Job drawing, mm, ordinate dimensions from the low corner. One solid piece. A direction names the side the tool comes from. Give positions to 0.01 mm unless a question says otherwise; leave off trailing zeros. Loops run counter-clockwise (first coordinate to the right, second up) from the corner with the lowest first, then second, coordinate; pieces in that order, holes last. Notation, with made-up numbers: M -8.75,-38.5 L 18.25,-38.5 A18 ccw 18.25,-5.5 Z; hole C 11.5,86.5 d7. An arc over 180 degrees is marked long. Put each result on its own line as item: value.
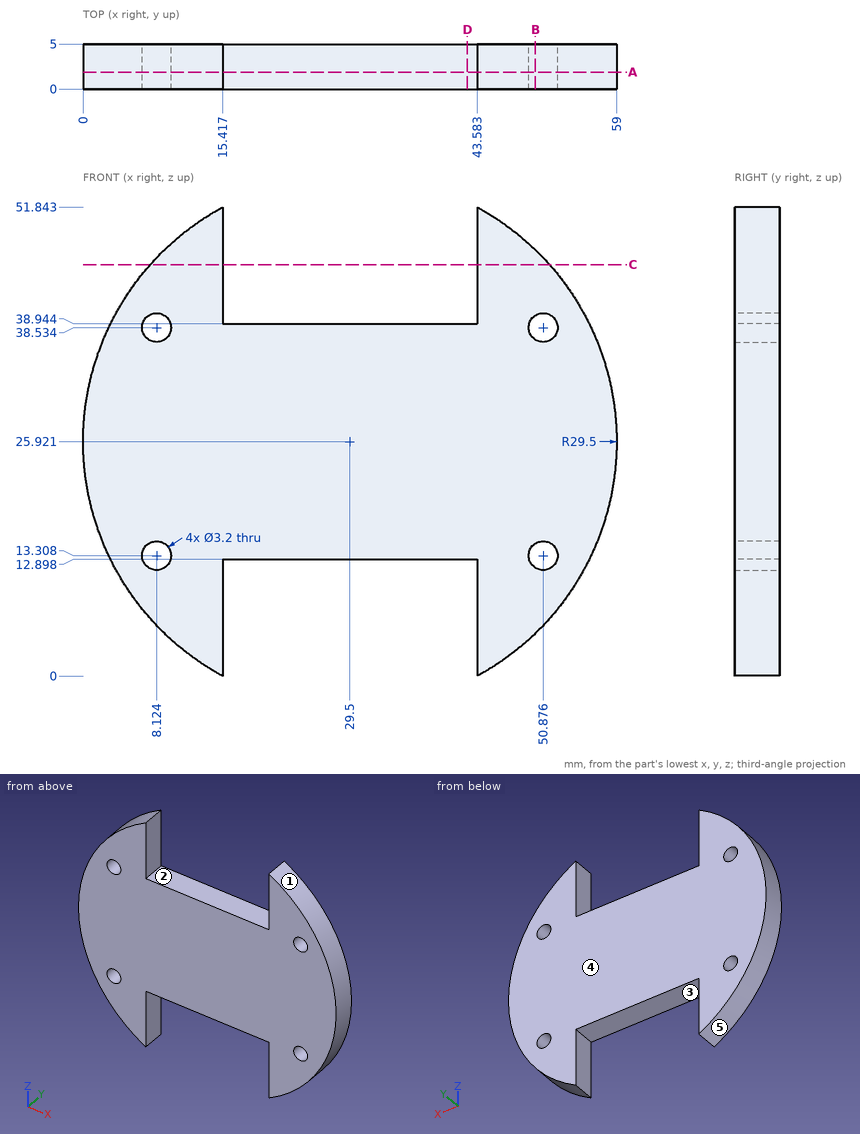
Q1. Probe line 1 (X direction, y = 0.75, z = 13) (1 decimal); line 2 (Z direction, x = 7, y = 2.5) (1 decimal); line 3 (X direction, y = 1.9, z = 12.5) (1 decimal). List the from-to ranges inside material, lowest first. Write a range as from..to.
Here are the results:
line 1: 3..6.6, 9.7..49.3, 52.4..56
line 2: 6.8..12.2, 14.4..37.4, 39.7..45
line 3: 3.2..6.7, 9.5..15.4, 43.6..49.5, 52.3..55.8
Q2. Drop flat-ended pins along their axis: pin 1 Ø2.5 at (y, z) = (3, 4.5) entering from -X (1 decimal); pin 2 Ø2 at (y, z) = (1, 16) entering from +X; pin 3 Ø2.5 at (y, z) = (3.5, 44.5) entering from +X (1 decimal). Give the stop position or say it passes through.
Here are the results:
pin 1: x = 8
pin 2: x = 57.62
pin 3: x = 53.4
Q3. Slice it at A-A (y = 1.9). List the corners of the cut face in (x, z) (1 decimal), and give its area (3 significant figures).
Here are the results:
outline: M 15.4,0 L 15.4,12.9 L 43.6,12.9 L 43.6,0 A29.5 ccw 43.6,51.8 L 43.6,38.9 L 15.4,38.9 L 15.4,51.8 A29.5 ccw Z; hole C 8.1,13.3 d3.2; hole C 8.1,38.5 d3.2; hole C 50.9,13.3 d3.2; hole C 50.9,38.5 d3.2
area: 1,840 mm²
Q4. Slice it at B-B (x = 50). List the corners of the cut face in (y, z) (1 decimal).
Here are the results:
outline: M 0,4.7 L 5,4.7 L 5,12 L 0,12 Z; M 0,14.6 L 5,14.6 L 5,37.2 L 0,37.2 Z; M 0,39.9 L 5,39.9 L 5,47.1 L 0,47.1 Z
Q5. Mould opens along X. For the marked faces 3, 4 and 5 say: pulls with the +X half, pulls with the -X half, needs draft (parallel to the pull), parting line crosses it, or undercut.
Here are the results:
face 3: undercut
face 4: needs draft
face 5: pulls with the -X half
Q6. Tool access for the marked faces 1 and 2: list every direction of +Z, -Z, +X, -X, +Y, -Y with a clear straight run to the whole face (end or side of a thin tool).
Here are the results:
face 1: +X, +Y, -Y
face 2: +Z, +Y, -Y
Q7. Slice it at C-C (z = 45.5). List the corners of the cut face in (x, y).
Here are the results:
outline: M 7.43,0 L 15.42,0 L 15.42,5 L 7.43,5 Z; M 43.58,0 L 51.57,0 L 51.57,5 L 43.58,5 Z
Q8. Slice it at D-D (x = 42.5). List the corners of the cut face in (y, z) (1 decimal).
Here are the results:
outline: M 0,12.9 L 5,12.9 L 5,38.9 L 0,38.9 Z
